Input: part model. Units: mm. Frame: model coordinates. A direction names the side the tool comes from. Give positions to 0.01 mm unless a question says otherwise; leave off trailing zeros. Loops run counter-clockwise (first coordinate to the right, second up) from the corner with the lowest first, then second, coordinate; pieces in that order, holes last. Notation, with made-up numbers: (34.5, 71) -> (58.5, 71) arc R26 cw to (58.5, 110) -> close; hole circle Ø2 at (18.25, -32). An arc over 180 degrees is marked (long way). Answer in a Markdown table with one row per item. Add a question column.
```python
from build123d import *

# Parameters (mm, degrees)
SKETCH1_W             = 30
SKETCH1_H             = 30
BOSS_EXTRUDE1_DEPTH   = 10
SKETCH2_R             = 14
CUT_EXTRUDE1_DEPTH    = 9
CUT_EXTRUDE2_DEPTH    = 44.370496884
F_3_0MM_DOWEL_HOLE1_D = 3
CUT_EXTRUDE3_DEPTH    = 7.25
FILLET1_R             = 3.5


with BuildPart() as part:
    # Sketch1 → Boss-Extrude1 (new body)
    with BuildSketch(Plane.XY):
        with Locations((15, 15)):
            Rectangle(SKETCH1_W, SKETCH1_H)
    extrude(amount=BOSS_EXTRUDE1_DEPTH)

    # Sketch2 → Cut-Extrude1 (cut)
    with BuildSketch(Plane.XY.offset(10)):
        with Locations((15, 15)):
            Circle(SKETCH2_R)
    extrude(amount=-CUT_EXTRUDE1_DEPTH, mode=Mode.SUBTRACT)

    # Sketch3 → Cut-Extrude2 (cut, through all)
    with BuildSketch(Plane.XY.offset(1)):
        with BuildLine():
            Line((14, 23.239538822), (14, 29.05542131))
            ThreePointArc((14, 29.05542131), (2.79687945, 22.045474934), (2.327648085, 8.838314749))
            Line((2.327648085, 8.838314749), (7.364350065, 11.746255993))
            ThreePointArc((7.364350065, 11.746255993), (7.811989149, 19.15), (14, 23.239538822))
        make_face()
        with BuildLine():
            Line((16, 23.239538822), (16, 29.05542131))
            ThreePointArc((16, 29.05542131), (27.20312055, 22.045474934), (27.672351915, 8.838314749))
            Line((27.672351915, 8.838314749), (22.635649935, 11.746255993))
            ThreePointArc((22.635649935, 11.746255993), (22.188010851, 19.15), (16, 23.239538822))
        make_face()
        with BuildLine():
            Line((21.635649935, 10.014205185), (26.672351915, 7.106263941))
            ThreePointArc((26.672351915, 7.106263941), (15, 0.909050131), (3.327648085, 7.106263941))
            Line((3.327648085, 7.106263941), (8.364350065, 10.014205185))
            ThreePointArc((8.364350065, 10.014205185), (15, 6.7), (21.635649935, 10.014205185))
        make_face()
    extrude(amount=-CUT_EXTRUDE2_DEPTH, mode=Mode.SUBTRACT)

    # Ø3.0mm Dowel Hole1 (through all)
    with Locations(Plane(origin=(0, 0, 0), x_dir=(-1, 0, 0), z_dir=(0, 0, -1))):
        with Locations((-27.5, 27.5), (-2.5, 27.5), (-2.5, 2.5), (-27.5, 2.5)):
            Hole(F_3_0MM_DOWEL_HOLE1_D / 2)

    # Sketch6 → Cut-Extrude3 (cut)
    with BuildSketch(Plane.XY.offset(10)):
        Polygon((9, 30), (6.267766953, 27.267766953), (3.535533906, 30), align=None)
        Polygon((23.732233047, 27.267766953), (26.464466094, 30), (21, 30), align=None)
        Polygon((30, 26.464466094), (30, 21), (27.267766953, 23.732233047), align=None)
        Polygon((30, 9), (30, 3.535533906), (27.267766953, 6.267766953), align=None)
        Polygon((26.464466094, 0), (21, 0), (23.732233047, 2.732233047), align=None)
        Polygon((9, 0), (3.535533906, 0), (6.267766953, 2.732233047), align=None)
        Polygon((0, 3.535533906), (0, 9), (2.732233047, 6.267766953), align=None)
        Polygon((0, 21), (0, 26.464466094), (2.732233047, 23.732233047), align=None)
    extrude(amount=-CUT_EXTRUDE3_DEPTH, mode=Mode.SUBTRACT)

    # Fillet1
    fillet1_edges = [part.edges().sort_by_distance(p)[0] for p in [
        (0, 30, 5),
        (30, 30, 5),
        (30, 0, 5),
        (0, 0, 5),
    ]]
    fillet(fillet1_edges, radius=FILLET1_R)


solid = part.part
```
1) Section A-A on x = 15. Output: boundary loops of the cut face in (y, z), and give its area (3 significant figures).
2) Pull-direction query (Y, two-part tool) for faces 6 (the face through (28.95, 1, 5.07)), 7 (the face through (8, 29, 6)), 8 (the face through (6, 29, 2.75)), 9 (the face through (29, 22, 6)); classes: +Y half, -Y half, draft (parallel to the pull), parting line (faces both ways), or undercut.
3) Section D-D on x = 24.5. Output: boundary loops of the cut face in (y, z), and give its area (3 significant figures).
4) Section C-C on z = 2. Output: boundary loops of the cut face in (x, y), and give its area (3 significant figures).
5) Pin query (flat end, axial travel): pin 1 (0.8 mm diameter, centred on x = 1, y = 6, fed in from +Z); pin 2 (1.5 mm diameter, centred on y = 7.5, z = 6, fed in from +X); pin 3 (12 mm diameter, centred on x = 18, y = 8.5, fed in from +Z). Return the tip coordinate at first contact, or that it passes through.
6) Material intervals for line 1 along Y through (x, z) = (3, 3.75); line 2 along Y through (x, z) = (2.5, 2.5); line 3 along Y through (x, z) = (5.25, 0.75), sorted ascending.
7) Section B-B on y = 15. Output: boundary loops of the cut face in (x, z).
8) Reachability of faces 1 (the face through (1, 22, 6)), 2 (the face through (4.921, 28.615, 6.426)), 3 (the face through (29, 8, 6)), 4 (the face through (25.079, 1.385, 6.426)), 5 (the face through (26, 2.57, 5.07)) from +Z, -Z, +X, -X, +Y, -Y: full face, straight path, thin tool, end or side. Return the list, or none.
Working result:
| question | item | result |
|---|---|---|
| 1 | outline | (0, 0) -> (0.91, 0) -> (0.91, 1) -> (1, 1) -> (1, 10) -> (0, 10) -> close; (6.7, 0) -> (30, 0) -> (30, 10) -> (29, 10) -> (29, 1) -> (6.7, 1) -> close |
| 1 | area | 42.2 mm2 |
| 2 | face 6 | -Y half |
| 2 | face 7 | +Y half |
| 2 | face 8 | draft |
| 2 | face 9 | undercut |
| 3 | outline | (0, 0) -> (4.59, 0) -> (4.59, 1) -> (4.72, 1) -> (4.72, 10) -> (1.96, 10) -> (1.96, 2.75) -> (0, 2.75) -> close; (8.36, 0) -> (10.67, 0) -> (10.67, 1) -> (8.36, 1) -> close; (25.28, 1) -> (25.41, 1) -> (25.41, 0) -> (30, 0) -> (30, 2.75) -> (28.04, 2.75) -> (28.04, 10) -> (25.28, 10) -> close |
| 3 | area | 67.9 mm2 |
| 4 | outline | (0, 3.5) arc R3.5 ccw to (3.5, 0) -> (26.5, 0) arc R3.5 ccw to (30, 3.5) -> (30, 26.5) arc R3.5 ccw to (26.5, 30) -> (3.5, 30) arc R3.5 ccw to (0, 26.5) -> close; hole circle Ø3 at (2.5, 2.5); hole circle Ø28 at (15, 15); hole circle Ø3 at (2.5, 27.5); hole circle Ø3 at (27.5, 2.5); hole circle Ø3 at (27.5, 27.5) |
| 4 | area | 245 mm2 |
| 5 | pin 1 | stops at z = 2.75 |
| 5 | pin 2 | stops at x = 29.25 |
| 5 | pin 3 | stops at z = 1 |
| 6 | line 1 | y = 0.04 to 1.09, 3.91 to 7.79, 22.21 to 26.09, 28.91 to 29.96 |
| 6 | line 2 | y = 0.15 to 1, 4 to 8.7, 21.3 to 26, 29 to 29.85 |
| 6 | line 3 | y = 0 to 4.83, 8.22 to 10.53, 25.17 to 30 |
| 7 | outline | (0, 0) -> (0.91, 0) -> (0.91, 1) -> (1, 1) -> (1, 10) -> (0, 10) -> close; (6.7, 0) -> (23.3, 0) -> (23.3, 1) -> (6.7, 1) -> close; (29, 1) -> (29.09, 1) -> (29.09, 0) -> (30, 0) -> (30, 10) -> (29, 10) -> close |
| 8 | face 1 | +Z, -X |
| 8 | face 2 | +Z, +Y |
| 8 | face 3 | +Z, +X |
| 8 | face 4 | +Z, -Y |
| 8 | face 5 | +Z, -Z |
